```python
from build123d import *

# Parameters (mm, degrees)
BOSS_EXTRUDE1_DEPTH = 76.2
SKETCH2_W           = 47.625
SKETCH2_H           = 50.8
CUT_EXTRUDE1_DEPTH  = 131.175
SKETCH3_W           = 47.625
SKETCH3_H           = 50.8
CUT_EXTRUDE2_DEPTH  = 131.175
FILLET1_R           = 5.08
FILLET2_R           = 12.7
SKETCH4_R           = 2.5
CUT_EXTRUDE3_DEPTH  = 132.982271537
SKETCH5_R           = 2.54
CUT_EXTRUDE4_DEPTH  = 132.982271537
CHAMFER1_SIZE       = 1.905
FILLET3_R           = 31.75


with BuildPart() as part:
    # Sketch1 → Boss-Extrude1 (new body)
    with BuildSketch(Plane(origin=(0, 0, 0), x_dir=(1, 0, 0), z_dir=(0, 1, 0))):
        Polygon((0, 76.2), (0, 0), (76.2, 0), (76.2, 3.175), (3.175, 3.175), (3.175, 76.2), align=None)
    extrude(amount=BOSS_EXTRUDE1_DEPTH)

    # Sketch2 → Cut-Extrude1 (cut, through all)
    with BuildSketch(Plane(origin=(0, 0, -3.175), x_dir=(-1, 0, 0), z_dir=(0, 0, -1))):
        with Locations((-52.3875, 50.8)):
            Rectangle(SKETCH2_W, SKETCH2_H)
    extrude(amount=-CUT_EXTRUDE1_DEPTH, mode=Mode.SUBTRACT)

    # Sketch3 → Cut-Extrude2 (cut, through all)
    with BuildSketch(Plane(origin=(3.175, 0, 0), x_dir=(0, 0, -1), z_dir=(1, 0, 0))):
        with Locations((52.3875, 50.8)):
            Rectangle(SKETCH3_W, SKETCH3_H)
    extrude(amount=-CUT_EXTRUDE2_DEPTH, mode=Mode.SUBTRACT)

    # Fillet1
    fillet1_edges = [part.edges().sort_by_distance(p)[0] for p in [
        (0, 38.1, 0),
    ]]
    fillet(fillet1_edges, radius=FILLET1_R)

    # Fillet2
    fillet2_edges = [part.edges().sort_by_distance(p)[0] for p in [
        (1.5875, 76.2, -28.575),
        (1.5875, 25.4, -76.2),
        (1.5875, 0, -76.2),
        (76.2, 0, -1.5875),
        (76.2, 25.4, -1.5875),
        (28.575, 76.2, -1.5875),
    ]]
    fillet(fillet2_edges, radius=FILLET2_R - 0.0001)  # a hair under: the kernel refuses the full size

    # Sketch4 → Cut-Extrude3 (cut, through all)
    with BuildSketch(Plane.XY):
        with Locations((63.5, 12.7)):
            Circle(SKETCH4_R)
        with Locations((19.685, 44.45)):
            Circle(SKETCH4_R)
    extrude(amount=-CUT_EXTRUDE3_DEPTH, mode=Mode.SUBTRACT)

    # Sketch5 → Cut-Extrude4 (cut, through all)
    with BuildSketch(Plane.ZY):
        with Locations((-63.5, 12.7)):
            Circle(SKETCH5_R)
        with Locations((-19.685, 63.5)):
            Circle(SKETCH5_R)
    extrude(amount=-CUT_EXTRUDE4_DEPTH, mode=Mode.SUBTRACT)

    # Chamfer1
    chamfer1_edges = [part.edges().sort_by_distance(p)[0] for p in [
        (0, 63.5, -22.225),
        (61, 12.7, 0),
        (17.185, 44.45, 0),
        (0, 12.7, -66.04),
    ]]
    chamfer(chamfer1_edges, length=CHAMFER1_SIZE)

    # Fillet3
    fillet3_edges = [part.edges().sort_by_distance(p)[0] for p in [
        (28.575, 25.4, -1.5875),
        (1.5875, 25.4, -28.575),
    ]]
    fillet(fillet3_edges, radius=FILLET3_R)


solid = part.part
```
Verification items for the finished model (mm, model axes). A direction names the side the tool comes from. Coordinates: 2 decimals unless noted, no trailing zeros. Loops run counter-clockwise (first coordinate to the right, second up) from the corner with the lowest first, then second, coordinate; pieces in that order, holes last. Notation, with made-up numbers: (-35, 26) -> (15, 26) arc R25 ccw to (15, 60) -> close; hole circle Ø10 at (-6, -5.5). An arc over 180 degrees is marked (long way). Put each result on its own line as item: value.
1. Section check D-D, the plane x = 32.5. Record the boundary of the cut face in (y, z) (3 decimals), then the cut area to 3 significant figures.
Result set:
outline: (0, -3.175) -> (41.858, -3.175) -> (41.858, 0) -> (0, 0) -> close
area: 133 mm^2
2. Section check B-B, the plane y = 55. Record the boundary of the cut face in (x, z) (3 decimals), then the cut area to 3 significant figures.
Result set:
outline: (0, -28.648) -> (3.175, -28.648) -> (3.175, -3.175) -> (28.648, -3.175) -> (28.648, 0) -> (5.08, 0) arc R5.08 ccw to (0, -5.08) -> close
area: 166 mm^2
3. Tool access check on faces 1 (the face through (2, 60, -28.575)), 2 (the face through (72.38, 3.62, -1.61)), 3 (the face through (28.575, 60, -2)). Record the directions out of +Z, -Z, +X, -X, +Y, -Y that give a thin tool (end or side, any length) a straight path to the whole face; none if there is none.
Result set:
face 1: -Z, +X, -X, +Y
face 2: +Z, -Z, +X, -Y
face 3: +Z, -Z, +X, +Y
4. Gauge pin test, flat ends, axial feed: P1, Ø8, axis at y = 63.5, z = -19.685, coming from the +X side (3 decimals); P2, Ø1.6, axis at x = 1.5, z = -61.5, coming from the +Y side; P3, Ø2, axis at x = 63.5, y = 12.5, coming from the +Z side; P4, Ø3.5, axis at x = 1, y = 61.5, coming from the -Z side (3 decimals). Record the tip position at first contact, or that the pin passes through.
Result set:
P1: stops at x = 3.175
P2: stops at y = 25.4
P3: passes through
P4: stops at z = -28.575
5. Thickness scan on line 1 (Y direction, x = 2, z = -63); line 2 (Z direction, x = 7, y = 33) (3 decimals); line 3 (X direction, y = 12, z = -2). Record the ranges inside material, lowest first.
Result set:
line 1: y = 0 to 10.21, 15.19 to 25.4
line 2: z = -3.175 to 0
line 3: x = 1.04 to 61.1, 65.9 to 76.18
6. Mould release check, pull along Z, two halves, no side actions. Record for faces 4 (the face through (2.531, 12.812, -66.038)), 5 (the face through (3.175, 29, -31)), 6 (the face through (1.565, 34.454, -38.123)): pulls with the +Z half, pulls with the -Z half, needs draft (parallel to the pull), parting line crosses it, or undercut.
Result set:
face 4: undercut
face 5: needs draft
face 6: pulls with the -Z half
7. Section check C-C, the plane z = -9.5. Record the boundary of the cut face in (x, y) (3 decimals), then the cut area to 3 significant figures.
Result set:
outline: (0, 0) -> (3.175, 0) -> (3.175, 76.2) -> (0, 76.2) -> close
area: 242 mm^2
8. Section check A-A, the plane y = 44.45. Record the boundary of the cut face in (x, z) (3 decimals).
Result set:
outline: (0, -31.226) -> (3.175, -31.226) -> (3.175, -3.175) -> (17.185, -3.175) -> (17.185, -1.905) -> (15.28, 0) -> (5.08, 0) arc R5.08 ccw to (0, -5.08) -> close; (22.185, -3.175) -> (31.226, -3.175) -> (31.226, 0) -> (24.09, 0) -> (22.185, -1.905) -> close
